Source: three-view drawing plus pictorial views. Frame: mm from the lowest corner of the part. Give positions to 0.01 mm unless a question says otherwise; leave off trailing zeros. Write each loop counter-clockwise with the first axis right and the second up, starting at its lowest first coordinate (ties: lowest second). Pieces come first, ordered by that corner, then holes. Notation, with made-up numbers: (26.25, 55.5) -> (74.25, 55.5) arc R19 cw to (74.25, 67.5) -> close; hole circle Ø5 at (42.5, 16.25). An arc over 180 degrees is marked (long way). Answer in a Markdown table with one row per item. Add a question column.
Item 1: Material intervals for probe 1 along X at (y, z) = (5, 460); probe 2 along Z at (x, y) = (250, 10.25); probe 3 along X at (y, z) = (13.5, 449.5), sorted ascending. Write a range as from..to.
Item 2: Section query C-C on x = 250. Output: boundary loops of the cut face in (y, z).
Item 3: Section query B-B on y = 9. Output: boundary loops of the cut face in (x, z).
Item 4: Section query A-A on z = 460. Output: boundary loops of the cut face in (x, y), plus the area to 3 significant figures.
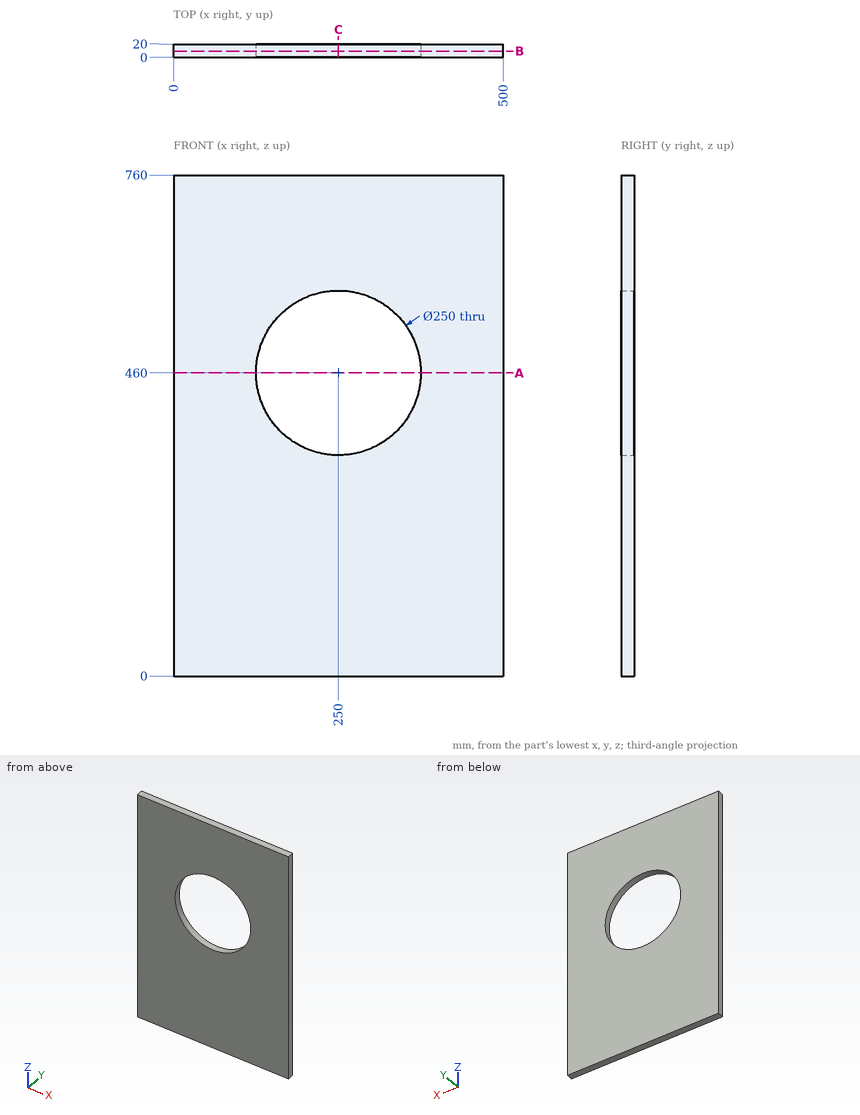
Findings below:
| question | item | result |
|---|---|---|
| 1 | probe 1 | x = 0..125, 375..500 |
| 1 | probe 2 | z = 0..335, 585..760 |
| 1 | probe 3 | x = 0..125.44, 374.56..500 |
| 2 | outline | (0, 0) -> (20, 0) -> (20, 335) -> (0, 335) -> close; (0, 585) -> (20, 585) -> (20, 760) -> (0, 760) -> close |
| 3 | outline | (0, 0) -> (500, 0) -> (500, 760) -> (0, 760) -> close; hole circle Ø250 at (250, 460) |
| 4 | outline | (0, 0) -> (125, 0) -> (125, 20) -> (0, 20) -> close; (375, 0) -> (500, 0) -> (500, 20) -> (375, 20) -> close |
| 4 | area | 5,000 mm^2 |
